```python
from build123d import *

# Parameters (mm, degrees)
SKETCH1_R                        = 3.175
BOSS_EXTRUDE1_DEPTH              = 57.15
F_10_0_1935_DIAMETER_HOLE1_D     = 4.9149
F_10_0_1935_DIAMETER_HOLE1_DEPTH = 54.61
F_10_0_1935_DIAMETER_HOLE1_TIP   = 1.476584928
SKETCH5_R                        = 3.937
SKETCH5_R_2                      = 3.175
BOSS_EXTRUDE2_DEPTH              = 2.54
FILLET1_R                        = 0.508
SKETCH6_R                        = 3.937
SKETCH6_R_2                      = 2.45745
BOSS_EXTRUDE3_DEPTH              = 27.94
CHAMFER1_SIZE                    = 0.508
FILLET2_R                        = 0.381


with BuildPart() as part:
    # Sketch1 → Boss-Extrude1 (new body)
    with BuildSketch(Plane(origin=(0, 0, 0), x_dir=(1, 0, 0), z_dir=(0, 1, 0))):
        Circle(SKETCH1_R)
    extrude(amount=BOSS_EXTRUDE1_DEPTH)

    # #10 (0.1935) Diameter Hole1
    with Locations(Plane.ZX.offset(57.15)):
        with Locations((0, 0)):
            Hole(F_10_0_1935_DIAMETER_HOLE1_D / 2, depth=F_10_0_1935_DIAMETER_HOLE1_DEPTH)
            with Locations((0, 0, -(F_10_0_1935_DIAMETER_HOLE1_DEPTH + F_10_0_1935_DIAMETER_HOLE1_TIP / 2))):  # 118° drill point
                Cone(0, F_10_0_1935_DIAMETER_HOLE1_D / 2, F_10_0_1935_DIAMETER_HOLE1_TIP, mode=Mode.SUBTRACT)

    # Sketch5 → Boss-Extrude2 (add)
    with BuildSketch(Plane(origin=(0, 57.15, 0), x_dir=(1, 0, 0), z_dir=(0, 1, 0))):
        Circle(SKETCH5_R)
        Circle(SKETCH5_R_2, mode=Mode.SUBTRACT)
    extrude(amount=-BOSS_EXTRUDE2_DEPTH)

    # Fillet1
    fillet1_edges = [part.edges().sort_by_distance(p)[0] for p in [
        (-3.175, 0, 0),
    ]]
    fillet(fillet1_edges, radius=FILLET1_R)

    # Sketch6 → Boss-Extrude3 (add)
    with BuildSketch(Plane(origin=(0, 57.15, 0), x_dir=(1, 0, 0), z_dir=(0, 1, 0))):
        Circle(SKETCH6_R)
        Circle(SKETCH6_R_2, mode=Mode.SUBTRACT)
    extrude(amount=BOSS_EXTRUDE3_DEPTH)

    # Chamfer1
    chamfer1_edges = [part.edges().sort_by_distance(p)[0] for p in [
        (-2.45745, 85.09, 0),
    ]]
    chamfer(chamfer1_edges, length=CHAMFER1_SIZE)

    # Fillet2
    fillet2_edges = [part.edges().sort_by_distance(p)[0] for p in [
        (-3.937, 85.09, 0),
    ]]
    fillet(fillet2_edges, radius=FILLET2_R)


solid = part.part
```
Could you check a few things on this model? Use its own coordinates, in mm. A direction names the side the tool comes from. Round coordinates to 2 decimals unless told otherwise and drop trailing zeros. Write each loop counter-clockwise with the first axis right and the second up, starting at its lowest first coordinate (ties: lowest second). Pieces come first, ordered by that corner, then holes. Notation, with made-up numbers: M 53,29.5 L 90,29.5 A14 cw 90,38.5 Z; hole C 19,49 d8. An arc over 180 degrees is marked long. Answer in a Markdown table with one row per item. Add a question column.
Q1. If we mould it in two halves opening along X, with no side actions, what happens to faces 1 (the conical face through (0.13, 1.32, 0.41)), 2 (the flat face through (0, 0, 0)), 3 (the cylindrical face through (-0.69, 27.18, 3.1))? For each: +X half, -X half, draft (parallel to the pull), parting line (faces both ways), or undercut.
Q2. If I drill on line 1 (Z direction, x = 0, y = 36) (3 decimals); line 2 (Z direction, x = 0, y = 71), over which ranges is the centre line in solid material (lowest first)? Write a range as from..to.
Q3. Imagine slicing it at A-A (y = 10.5). Please give me the cut outline in (x, z) (3 decimals).
Q4. On a 3-axis mill with a long thin cutter (end or side, diameter ignored), from which of +Z, -Z, +X, -X, +Y, -Y can I reach the whole of each face in a straight line? I mean faces 4 (the flat face through (-3, 54.61, -2)), 5 (the flat face through (1, 85.09, 3)). Say none if no direction works.
Q5. Will these pins go through, and if not, where does the flat tip stop? pin 1 Ø3 at (x, y) = (1.5, 16.5) entering from -Z (3 decimals); pin 2 Ø1.5 at (y, z) = (53, -1.5) entering from -X.
Values:
| question | item | result |
|---|---|---|
| 1 | face 1 | undercut |
| 1 | face 2 | draft |
| 1 | face 3 | parting line |
| 2 | line 1 | -3.175..-2.457, 2.457..3.175 |
| 2 | line 2 | -3.94..-2.46, 2.46..3.94 |
| 3 | outline | C 0,0 d6.35; hole C 0,0 d4.915 |
| 4 | face 4 | -Y |
| 4 | face 5 | +Z, -Z, +X, -X, +Y |
| 5 | pin 1 | z = -3.175 |
| 5 | pin 2 | x = -3.09 |
